Design review of the part built by this model. Coordinates are the model's own, in mm. A direction names the side the tool comes from. Give positions to 0.01 mm unless a question says otherwise; leave off trailing zeros. Order: outer loops, then holes, each group sorted by start corner. A loop starts at its lowest first (then second) coordinate and runs counter-clockwise, first axis right, second up. Notation, with made-up numbers: M -6.75,54.25 L 11.25,54.25 A32 ccw 11.25,87.25 Z; hole C -8,-13.5 d9. An arc over 180 degrees is marked long. Answer as a JSON object with one key per item and string values.
from build123d import *

# Parameters (mm, degrees)
SKETCH_1_W          = 143
SKETCH_1_H          = 72
EXTRUDE_1_DEPTH     = 2
SKETCH_2_R          = 1.5
CUT_EXTRUDE_1_DEPTH = 2
SKETCH_3_W          = 14.9
SKETCH_3_H          = 8
SKETCH_3_W_2        = 15
EXTRUDE_2_DEPTH     = 8
SKETCH_3_3_W        = 15.75
SKETCH_3_3_H        = 18
SKETCH_3_3_W_2      = 16.25
EXTRUDE_3_DEPTH     = 12
SKETCH_3_4_W        = 6.1
SKETCH_3_4_H        = 8
SKETCH_3_4_W_2      = 6
SKETCH_3_4_W_3      = 6.2
EXTRUDE_4_DEPTH     = 12


with BuildPart() as part:
    # 草图1 → 凸台-拉伸1 (new body)
    with BuildSketch(Plane.XY):
        with Locations((71.5, 36)):
            Rectangle(SKETCH_1_W, SKETCH_1_H)
    extrude(amount=EXTRUDE_1_DEPTH)

    # 草图2 → 切除-拉伸1 (cut)
    with BuildSketch(Plane(origin=(0, 0, 0), x_dir=(-1, 0, 0), z_dir=(0, 0, -1))):
        with Locations((-139.5, 68.5)):
            Circle(SKETCH_2_R)
        with Locations((-139.5, 3.5)):
            Circle(SKETCH_2_R)
        with Locations((-3.5, 68.5)):
            Circle(SKETCH_2_R)
        with Locations((-3.5, 3.5)):
            Circle(SKETCH_2_R)
    extrude(amount=-CUT_EXTRUDE_1_DEPTH, mode=Mode.SUBTRACT)

    # 草图3 → 凸台-拉伸2 (add)
    with BuildSketch(Plane.XY.offset(2)):
        with Locations((78.95, 7)):
            Rectangle(SKETCH_3_W, SKETCH_3_H)
        with Locations((63.95, 7)):
            Rectangle(SKETCH_3_W, SKETCH_3_H)
        with Locations((93.95, 7)):
            Rectangle(SKETCH_3_W, SKETCH_3_H)
        with Locations((48.95, 7)):
            Rectangle(SKETCH_3_W, SKETCH_3_H)
        with Locations((108.95, 7)):
            Rectangle(SKETCH_3_W, SKETCH_3_H)
        with Locations((33.95, 7)):
            Rectangle(SKETCH_3_W, SKETCH_3_H)
        with Locations((124, 7)):
            Rectangle(SKETCH_3_W_2, SKETCH_3_H)
        with Locations((18.95, 7)):
            Rectangle(SKETCH_3_W, SKETCH_3_H)
    extrude(amount=EXTRUDE_2_DEPTH)

    # 草图3<3> → 凸台-拉伸3 (add)
    with BuildSketch(Plane.XY.offset(2)):
        with Locations((79.375, 27)):
            Rectangle(SKETCH_3_3_W, SKETCH_3_3_H)
        with Locations((63.125, 27)):
            Rectangle(SKETCH_3_3_W, SKETCH_3_3_H)
        with Locations((95.625, 27)):
            Rectangle(SKETCH_3_3_W, SKETCH_3_3_H)
        with Locations((46.875, 27)):
            Rectangle(SKETCH_3_3_W, SKETCH_3_3_H)
        with Locations((111.875, 27)):
            Rectangle(SKETCH_3_3_W, SKETCH_3_3_H)
        with Locations((30.625, 27)):
            Rectangle(SKETCH_3_3_W, SKETCH_3_3_H)
        with Locations((128.375, 27)):
            Rectangle(SKETCH_3_3_W_2, SKETCH_3_3_H)
        with Locations((14.375, 27)):
            Rectangle(SKETCH_3_3_W, SKETCH_3_3_H)
    extrude(amount=EXTRUDE_3_DEPTH)

    # 草图3<4> → 凸台-拉伸4 (add)
    with BuildSketch(Plane.XY.offset(2)):
        with Locations((47.05, 65)):
            Rectangle(SKETCH_3_4_W, SKETCH_3_4_H)
        with Locations((53.1, 65)):
            Rectangle(SKETCH_3_4_W_2, SKETCH_3_4_H)
        with Locations((59.25, 65)):
            Rectangle(SKETCH_3_4_W, SKETCH_3_4_H)
        with Locations((65.3, 65)):
            Rectangle(SKETCH_3_4_W_2, SKETCH_3_4_H)
        Polygon((68.4, 69), (68.4, 61), (74.5, 61), (74.5, 69), (71.5, 69), align=None)
        with Locations((77.5, 65)):
            Rectangle(SKETCH_3_4_W_2, SKETCH_3_4_H)
        with Locations((83.65, 65)):
            Rectangle(SKETCH_3_4_W, SKETCH_3_4_H)
        with Locations((89.75, 65)):
            Rectangle(SKETCH_3_4_W, SKETCH_3_4_H)
        with Locations((95.9, 65)):
            Rectangle(SKETCH_3_4_W_3, SKETCH_3_4_H)
    extrude(amount=EXTRUDE_4_DEPTH)


solid = part.part
(1) Draft analysis for pull direction Y (two halves, no side actions). For faces 1 (the flat face through (34, 7, 10)), 2 (the cylindrical face through (2.694, 69.765, 0.986)), state which applies: +Y half, -Y half, draft (parallel to the pull), parting line (faces both ways), or undercut.
Checked values:
{"face 1": "draft", "face 2": "undercut"}
(2) We need section C-C (x = 94). Write out the cut boundary in (y, z), plus the area to 3 significant figures.
Checked values:
{"outline": "M 0,0 L 72,0 L 72,2 L 69,2 L 69,14 L 61,14 L 61,2 L 36,2 L 36,14 L 18,14 L 18,2 L 11,2 L 11,10 L 3,10 L 3,2 L 0,2 Z", "area": "520 mm^2"}
(3) We need section D-D (x = 109). Write out the cut boundary in (y, z), plus the area to 3 significant figures.
Checked values:
{"outline": "M 0,0 L 72,0 L 72,2 L 36,2 L 36,14 L 18,14 L 18,2 L 11,2 L 11,10 L 3,10 L 3,2 L 0,2 Z", "area": "424 mm^2"}
(4) To check wall thickness, follow L1, parallel to X at y = 68.5, z = 0.4; L2, parallel to Y at x = 3.5, z = 1.55; L3, parallel to Y at x = 60.5, z = 9.25. State the ranges of each line that lie inside material, in increasing order. Write a range as from..to.
Checked values:
{"L1": "x = 0..2, 5..138, 141..143", "L2": "y = 0..2, 5..67, 70..72", "L3": "y = 3..11, 18..36, 61..69"}
(5) Insertion check: pin 1 (6 mm diameter, centred on y = 30.5, z = 6, fed in from +X); pin 2 (2.5 mm diameter, centred on x = 111.5, z = 6.5, fed in from +Y); pin 3 (6 mm diameter, centred on x = 98, z = 8.5, fed in from +Y). Each pin has a flat end and moves straight along its axis. Give the tip position at first contact, or say it passes through.
Checked values:
{"pin 1": "stops at x = 136.5", "pin 2": "stops at y = 36", "pin 3": "stops at y = 69"}
(6) We need section A-A (x = 3.5). Write out the cut boundary in (y, z), plus the area to 3 significant figures.
Checked values:
{"outline": "M 0,0 L 2,0 L 2,2 L 0,2 Z; M 5,0 L 67,0 L 67,2 L 5,2 Z; M 70,0 L 72,0 L 72,2 L 70,2 Z", "area": "132 mm^2"}
(7) Tool access review of faces 3 (the flat face through (54.75, 27, 8)), 4 (the flat face through (90, 61, 8)), 5 (the flat face through (104, 27, 8)): name each direction out of +Z, -Z, +X, -X, +Y, -Y from which nothing blocks a thin tool from reaching the whole face with its end or side.
Checked values:
{"face 3": "+Z", "face 4": "+Z, +X, -X", "face 5": "+Z, +Y"}
(8) We need section B-B (z = 4.25). Count the separate pieces of the cut face and the enclosed holes in it, plus the area to 3 significant figures.
Checked values:
{"separate pieces": "20", "enclosed holes": "0", "area": "3,670 mm^2"}
